Geometry: final body of the model. Coordinates: model frame, mm. A direction names the side the tool comes from. Round coordinates to 2 decimals unless told otherwise and drop trailing zeros. Write each loop counter-clockwise with the first axis right and the second up, starting at its lowest first coordinate (ties: lowest second). Pieces come first, ordered by that corner, then holes. Notation, with made-up numbers: (0, 35) - (44, 35) arc R5 ccw to (44, 42) - close; hole circle Ø2 at (38.25, -17.75). An arc over 180 degrees is marked (long way). Write each question's results on one line, items separated by ' | '.
from build123d import *

# Parameters (mm, degrees)
SKETCH1_W               = 2
SKETCH1_H               = 1
SKETCH1_W_2             = 2.5
SKETCH1_H_2             = 23
CUT_EXTRUDE1_REACH      = 38.197
CUT_EXTRUDE1_END_RADIUS = 10


with BuildPart() as part:
    # Sketch1 → Revolve1 (revolve)
    with BuildSketch(Plane.XY, mode=Mode.PRIVATE) as revolve1_sk:
        with BuildLine():
            Line((0, 20.5), (0, 18.9))
            ThreePointArc((0, 18.9), (5.024937811, 16.693186096), (6.8, 11.5))
            Line((6.8, 11.5), (8, 11.5))
            Line((8, 11.5), (8, 12.5))
            ThreePointArc((8, 12.5), (5.656854249, 18.156854249), (0, 20.5))
        make_face()
        with Locations((9, 12)):
            Rectangle(SKETCH1_W, SKETCH1_H)
        with Locations((11.25, 11.5)):
            Rectangle(SKETCH1_W_2, SKETCH1_H_2)
    revolve(revolve1_sk.sketch.rotate(Axis((0, 0, 0), (0, 1, 0)), 90), axis=Axis((0, 0, 0), (0, 1, 0)))

    # Cut-Extrude1: up to this cylinder (the profile starts outside it)
    cut_extrude1_end = Plane(origin=(0, 11.5, 0), z_dir=(0, -1, 0)) * Cylinder(CUT_EXTRUDE1_END_RADIUS, 111.394, mode=Mode.PRIVATE)
    # Sketch2 → Cut-Extrude1 (cut, up to the surface)
    with BuildSketch(Plane(origin=(12.5, 0, 0), x_dir=(0, 0, -1), z_dir=(1, 0, 0)), mode=Mode.PRIVATE) as cut_extrude1_sk1:
        with BuildLine():
            ThreePointArc((0, 19.1), (-0.6, 18.5), (0, 17.9))
            Line((0, 17.9), (0, 19.1))
        make_face()
    cut_extrude1_tool1 = extrude(cut_extrude1_sk1.sketch, amount=-CUT_EXTRUDE1_REACH, mode=Mode.PRIVATE) - cut_extrude1_end
    add(cut_extrude1_tool1.solids().sort_by_distance((12.5, 18.5, 0.254648))[0], mode=Mode.SUBTRACT)
    # Sketch2 → Cut-Extrude1 (cut, up to the surface)
    with BuildSketch(Plane(origin=(12.5, 0, 0), x_dir=(0, 0, -1), z_dir=(1, 0, 0)), mode=Mode.PRIVATE) as cut_extrude1_sk2:
        with BuildLine():
            Line((0, 19.1), (0, 17.9))
            ThreePointArc((0, 17.9), (0.424264069, 18.075735931), (0.6, 18.5))
            ThreePointArc((0.6, 18.5), (0.424264069, 18.924264069), (0, 19.1))
        make_face()
    cut_extrude1_tool2 = extrude(cut_extrude1_sk2.sketch, amount=-CUT_EXTRUDE1_REACH, mode=Mode.PRIVATE) - cut_extrude1_end
    add(cut_extrude1_tool2.solids().sort_by_distance((12.5, 18.5, -0.254648))[0], mode=Mode.SUBTRACT)
    # Sketch2 → Cut-Extrude1 (cut, up to the surface)
    with BuildSketch(Plane(origin=(12.5, 0, 0), x_dir=(0, 0, -1), z_dir=(1, 0, 0)), mode=Mode.PRIVATE) as cut_extrude1_sk3:
        with BuildLine():
            ThreePointArc((0, 19.1), (-0.6, 18.5), (0, 17.9))
            Line((0, 17.9), (0, 19.1))
        make_face()
    cut_extrude1_tool3 = extrude(cut_extrude1_sk3.sketch, amount=-CUT_EXTRUDE1_REACH, mode=Mode.PRIVATE) - cut_extrude1_end
    add(cut_extrude1_tool3.solids().sort_by_distance((12.5, 18.5, 0.254648))[0], mode=Mode.SUBTRACT)
    # Sketch2 → Cut-Extrude1 (cut, up to the surface)
    with BuildSketch(Plane(origin=(12.5, 0, 0), x_dir=(0, 0, -1), z_dir=(1, 0, 0)), mode=Mode.PRIVATE) as cut_extrude1_sk4:
        with BuildLine():
            Line((0, 19.1), (0, 17.9))
            ThreePointArc((0, 17.9), (0.424264069, 18.075735931), (0.6, 18.5))
            ThreePointArc((0.6, 18.5), (0.424264069, 18.924264069), (0, 19.1))
        make_face()
    cut_extrude1_tool4 = extrude(cut_extrude1_sk4.sketch, amount=-CUT_EXTRUDE1_REACH, mode=Mode.PRIVATE) - cut_extrude1_end
    add(cut_extrude1_tool4.solids().sort_by_distance((12.5, 18.5, -0.254648))[0], mode=Mode.SUBTRACT)
    # Sketch2 → Cut-Extrude1 (cut, up to the surface)
    with BuildSketch(Plane(origin=(12.5, 0, 0), x_dir=(0, 0, -1), z_dir=(1, 0, 0)), mode=Mode.PRIVATE) as cut_extrude1_sk5:
        with BuildLine():
            ThreePointArc((0, 5.1), (-0.6, 4.5), (0, 3.9))
            Line((0, 3.9), (0, 5.1))
        make_face()
    cut_extrude1_tool5 = extrude(cut_extrude1_sk5.sketch, amount=-CUT_EXTRUDE1_REACH, mode=Mode.PRIVATE) - cut_extrude1_end
    add(cut_extrude1_tool5.solids().sort_by_distance((12.5, 4.5, 0.254648))[0], mode=Mode.SUBTRACT)
    # Sketch2 → Cut-Extrude1 (cut, up to the surface)
    with BuildSketch(Plane(origin=(12.5, 0, 0), x_dir=(0, 0, -1), z_dir=(1, 0, 0)), mode=Mode.PRIVATE) as cut_extrude1_sk6:
        with BuildLine():
            Line((0, 5.1), (0, 3.9))
            ThreePointArc((0, 3.9), (0.424264069, 4.075735931), (0.6, 4.5))
            ThreePointArc((0.6, 4.5), (0.424264069, 4.924264069), (0, 5.1))
        make_face()
    cut_extrude1_tool6 = extrude(cut_extrude1_sk6.sketch, amount=-CUT_EXTRUDE1_REACH, mode=Mode.PRIVATE) - cut_extrude1_end
    add(cut_extrude1_tool6.solids().sort_by_distance((12.5, 4.5, -0.254648))[0], mode=Mode.SUBTRACT)
    # Sketch2 → Cut-Extrude1 (cut, up to the surface)
    with BuildSketch(Plane(origin=(12.5, 0, 0), x_dir=(0, 0, -1), z_dir=(1, 0, 0)), mode=Mode.PRIVATE) as cut_extrude1_sk7:
        with BuildLine():
            ThreePointArc((0, 5.1), (-0.6, 4.5), (0, 3.9))
            Line((0, 3.9), (0, 5.1))
        make_face()
    cut_extrude1_tool7 = extrude(cut_extrude1_sk7.sketch, amount=-CUT_EXTRUDE1_REACH, mode=Mode.PRIVATE) - cut_extrude1_end
    add(cut_extrude1_tool7.solids().sort_by_distance((12.5, 4.5, 0.254648))[0], mode=Mode.SUBTRACT)
    # Sketch2 → Cut-Extrude1 (cut, up to the surface)
    with BuildSketch(Plane(origin=(12.5, 0, 0), x_dir=(0, 0, -1), z_dir=(1, 0, 0)), mode=Mode.PRIVATE) as cut_extrude1_sk8:
        with BuildLine():
            Line((0, 5.1), (0, 3.9))
            ThreePointArc((0, 3.9), (0.424264069, 4.075735931), (0.6, 4.5))
            ThreePointArc((0.6, 4.5), (0.424264069, 4.924264069), (0, 5.1))
        make_face()
    cut_extrude1_tool8 = extrude(cut_extrude1_sk8.sketch, amount=-CUT_EXTRUDE1_REACH, mode=Mode.PRIVATE) - cut_extrude1_end
    add(cut_extrude1_tool8.solids().sort_by_distance((12.5, 4.5, -0.254648))[0], mode=Mode.SUBTRACT)


solid = part.part
Q1. Section query B-B, the plane y = 14.5. Return loops of the section in (x, z), plus the area to 3 significant figures.
Answer block:
outline: circle Ø25 at (0, 0); circle Ø15.49 at (0, 0); hole circle Ø20 at (0, 0); hole circle Ø12.76 at (0, 0) | area: 237 mm2
Q2. Ray query, line 1 along X through (y, z) = (16.5, 0); line 2 along Z through (x, y) = (-5, 13.25); line 3 along X through (y, z) = (7.5, 0). Return the intervals inside material, ascending.
Answer block:
line 1: -12.5 to -10, -6.93 to -5.2, 5.2 to 6.93, 10 to 12.5 | line 2: -11.46 to -8.66, -6.2 to -4.49, 4.49 to 6.2, 8.66 to 11.46 | line 3: -12.5 to -10, 10 to 12.5
Q3. Access query for faces 1 (the flat face through (2, 11.5, 7)), 2 (the cylindrical face through (0, 18, 10)), 3 (the flat face through (-10.2, 0, -0.1)). Directions: +Z, -Z, +X, -X, +Y, -Y. A direction counts if a zero-diameter tool reaches every point of the face in a straight line with its end or side. Return the directions, or none.
Answer block:
face 1: -Y | face 2: +Y | face 3: +Z, -Z, +X, -X, -Y
Q4. Section query C-C, the plane z = -7.25. Return loops of the section in (x, y).
Answer block:
outline: (-10.18, 0) - (-6.89, 0) - (-6.89, 11.5) - (6.89, 11.5) - (6.89, 0) - (10.18, 0) - (10.18, 23) - (6.89, 23) - (6.89, 12.5) - (3.38, 12.5) arc R3.38 ccw to (-3.38, 12.5) - (-6.89, 12.5) - (-6.89, 23) - (-10.18, 23) - close
Q5. Section query A-A, the plane x = 0. Return loops of the section in (y, z), plus the area to 3 significant figures.
Answer block:
outline: (0, -12.5) - (23, -12.5) - (23, -10) - (12.5, -10) - (12.5, -8) arc R8 ccw to (12.5, 8) - (12.5, 10) - (23, 10) - (23, 12.5) - (0, 12.5) - (0, 10) - (11.5, 10) - (11.5, 6.8) arc R6.82 cw (long way) to (11.5, -6.8) - (11.5, -10) - (0, -10) - close | area: 155 mm2
Q6. Pin query (flat end, axial travel): pin 1 (1.5 mm diameter, centred on x = 7, y = 18, fed in from -Z); pin 2 (4 mm diameter, centred on y = 14, z = -4, fed in from -X); pin 3 (1 mm diameter, centred on x = 9, y = 20.5, fed in from +Z). Return the tip coordinate at first contact, or that it passes through.
Answer block:
pin 1: z = -10.83 | pin 2: x = -12.34 | pin 3: z = 9.17
Q7. Section query D-D, the plane y = 10.25. Return loops of the section in (x, z).
Answer block:
outline: circle Ø25 at (0, 0); hole circle Ø20 at (0, 0)
Q8. Mould query, pull axis X, two halves, no side actions, for faces 4 (the cylindrical face through (-3.755, 11.661, -11.923)), 5 (the flat face through (-8.2, 12.5, 0)), 6 (the flat face through (-10.2, 23, -0.1)). Classes: pulls with the +X half, pulls with the -X half, needs draft (parallel to the pull), parting line crosses it, or undercut.
Answer block:
face 4: parting line crosses it | face 5: undercut | face 6: needs draft
